from build123d import *

# Parameters (mm, degrees)
F0_W     = 70
F0_H     = 30
F1_DEPTH = 70
F2_R     = 10
F3_DEPTH = 30.001
F4_R     = 12.7
F5_SIZE  = 25.4


with BuildPart() as f1:
    # F0 (on Front) → F1 (new body)
    with BuildSketch(Plane.XZ):
        Rectangle(F0_W, F0_H)
    extrude(amount=F1_DEPTH)

    # F2 (on face) → F3 (cut, through all)
    with BuildSketch(Plane.XY.offset(15)):
        with Locations((0, -35)):
            Circle(F2_R)
    extrude(amount=-F3_DEPTH, mode=Mode.SUBTRACT)

    # F4
    f4_edges = [f1.edges().sort_by_distance(p)[0] for p in [
        (-35, 0, 0),
        (35, 0, 0),
    ]]
    fillet(f4_edges, radius=F4_R)

    # F5
    f5_edges = [f1.edges().sort_by_distance(p)[0] for p in [
        (-35, -70, 0),
        (35, -70, 0),
    ]]
    chamfer(f5_edges, length=F5_SIZE)


solid = f1.part
Design review of the part built by this model. Coordinates are the model's own, in mm. Coordinates: 2 decimals unless noted, no trailing zeros. Loops run counter-clockwise (first coordinate to the right, second up) from the corner with the lowest first, then second, coordinate; pieces in that order, holes last. Notation, with made-up numbers: (58, 80) - (72, 80) arc R26 ccw to (72, 95) - close; hole circle Ø5 at (-5.5, -32). An arc over 180 degrees is marked (long way). Use CSV: the item, a comma, the result in double quotes. Start each with the question number.
1. To check wall thickness, follow probe 1 along Y at (x, z) = (0, 6.5); probe 2 along Y at (x, z) = (2, -0.75); probe 3 along X at (y, z) = (-41, 10.75). State the ranges of each line that lie inside material, in increasing order.
2. Add section C-C on x = 0. Give the boundary of the cut face in (y, z).
3. Add section D-D on y = -50.5. Give the boundary of the cut face in (x, z).
4. Mouldability with a two-part tool opening along Y and no side actions: class faces 1 (the flat face through (-22.1, -57.5, -0.2)), 2 (the flat face through (0, 0, 0)), 3 (the cylindrical face through (-2.17, -44.76, 0.21)) as released by +Y, released by -Y, zero draft, split by the parting line, or undercut.
5. Add section A-A on y = -35. Give the boundary of the cut face in (x, z).
6. Clearance check with flat-ended pins moving along their axes: pin 1 (5 mm diameter, centred on y = -9.5, z = 4, fed in from +X); pin 2 (6 mm diameter, centred on x = 25, y = -59.5, fed in from +Z). State where each tip first meets the part, or that it passes through.
7. Add section B-B on z = -12.75. Give the boundary of the cut face in (x, y).
Resolved:
1,probe 1,"-70 to -45, -25 to 0"
1,probe 2,"-70 to -44.8, -25.2 to 0"
1,probe 3,"-35 to -8, 8 to 35"
2,outline,"(-70, -15) - (-45, -15) - (-45, 15) - (-70, 15) - close; (-25, -15) - (0, -15) - (0, 15) - (-25, 15) - close"
3,outline,"(-29.1, -15) - (29.1, -15) - (29.1, 15) - (-29.1, 15) - close"
4,face 1,"released by -Y"
4,face 2,"released by +Y"
4,face 3,"undercut"
5,outline,"(-35, -15) - (-10, -15) - (-10, 15) - (-35, 15) - close; (10, -15) - (35, -15) - (35, 15) - (10, 15) - close"
6,pin 1,"x = 34.98"
6,pin 2,"through"
7,outline,"(-35, -44.6) - (-9.6, -70) - (9.6, -70) - (35, -44.6) - (35, -12.7) arc R12.7 ccw to (22.3, 0) - (-22.3, 0) arc R12.7 ccw to (-35, -12.7) - close; hole circle Ø20 at (0, -35)"
